from build123d import *

# Parameters (mm, degrees)
SKETCH_1_W      = 23
SKETCH_1_H      = 20
SKETCH_1_R      = 0.5
SKETCH_1_R_2    = 1.5
EXTRUDE_1_DEPTH = 2
SKETCH_2_R      = 3
SKETCH_2_R_2    = 1.5
EXTRUDE_2_DEPTH = 4


with BuildPart() as part:
    # 草图1 → 凸台-拉伸1 (new body)
    with BuildSketch(Plane.XY):
        Rectangle(SKETCH_1_W, SKETCH_1_H)
        with Locations((-8.5, 9)):
            Circle(SKETCH_1_R, mode=Mode.SUBTRACT)
        with Locations((-7.803030303, -9)):
            Circle(SKETCH_1_R, mode=Mode.SUBTRACT)
        with Locations((9.5, 0)):
            Circle(SKETCH_1_R, mode=Mode.SUBTRACT)
        with Locations((2.5, 8)):
            Circle(SKETCH_1_R, mode=Mode.SUBTRACT)
        with Locations((2.5, -8)):
            Circle(SKETCH_1_R, mode=Mode.SUBTRACT)
        with Locations((5.5, 0)):
            Circle(SKETCH_1_R_2, mode=Mode.SUBTRACT)
    extrude(amount=EXTRUDE_1_DEPTH)

    # 草图2 → 凸台-拉伸2 (add)
    with BuildSketch(Plane.XY.offset(2)):
        with Locations((5.5, 0)):
            Circle(SKETCH_2_R)
        with Locations((5.5, 0)):
            Circle(SKETCH_2_R_2, mode=Mode.SUBTRACT)
    extrude(amount=EXTRUDE_2_DEPTH)


solid = part.part
Source: CAD feature listing. Evaluate the final solid. Frame: model axes, mm. Coordinates: 2 decimals unless noted, no trailing zeros. Loops run counter-clockwise (first coordinate to the right, second up) from the corner with the lowest first, then second, coordinate; pieces in that order, holes last. Notation, with made-up numbers: M -38.5,33 L 0.5,33 A16 cw 0.5,56 Z; hole C 87,5 d1. An arc over 180 degrees is marked long. Answer in a Markdown table with one row per item.
Q1. Section A-A on y = 0. Return the cut outline in (x, z).
Answers below:
| item | result |
|---|---|
| outline | M -11.5,0 L 4,0 L 4,6 L 2.5,6 L 2.5,2 L -11.5,2 Z; M 7,0 L 9,0 L 9,2 L 8.5,2 L 8.5,6 L 7,6 Z; M 10,0 L 11.5,0 L 11.5,2 L 10,2 Z |
Q2. Section C-C on y = -9. Return the cut outline in (x, z).
Answers below:
| item | result |
|---|---|
| outline | M -11.5,0 L -8.3,0 L -8.3,2 L -11.5,2 Z; M -7.3,0 L 11.5,0 L 11.5,2 L -7.3,2 Z |
Q3. Section D-D on z = 0.8. Return the cut outline in (x, y).
Answers below:
| item | result |
|---|---|
| outline | M -11.5,-10 L 11.5,-10 L 11.5,10 L -11.5,10 Z; hole C -8.5,9 d1; hole C -7.8,-9 d1; hole C 2.5,-8 d1; hole C 2.5,8 d1; hole C 5.5,0 d3; hole C 9.5,0 d1 |
Q4. First-contact query: pin 1 (2.5 mm diameter, centred on x = 5.5, y = 0, fed in from -Z); pin 2 (3 mm diameter, centred on x = -2, y = -0.5, fed in from +Z). Flat tips, straight axial feed; report the tip coordinate or a pass-through.
Answers below:
| item | result |
|---|---|
| pin 1 | passes through |
| pin 2 | stops at z = 2 |
Q5. Draft query along Y for faces 1 (the cylindrical face through (4.3, -0.9, 3)), 2 (the cylindrical face through (9, 0, 1)), 3 (the flat face through (0, -10, 1)), 4 (the cylindrical face through (8.27, -1.15, 3.97)). Return one class per face: pulls with the +Y half, pulls with the -Y half, needs draft (parallel to the pull), parting line crosses it, or undercut.
Answers below:
| item | result |
|---|---|
| face 1 | undercut |
| face 2 | undercut |
| face 3 | pulls with the -Y half |
| face 4 | parting line crosses it |
Q6. Ray query, probe 1 along Y at (x, z) = (2.5, 1.05); probe 2 along Y at (x, z) = (5.5, 3.1); probe 3 along Z at (x, y) = (-3.5, 2.5). Return the intervals inside material, ascending. Write a range as from..to.
Answers below:
| item | result |
|---|---|
| probe 1 | y = -10..-8.5, -7.5..7.5, 8.5..10 |
| probe 2 | y = -3..-1.5, 1.5..3 |
| probe 3 | z = 0..2 |
Q7. Section B-B on x = 5.5. Return the cut outline in (y, z).
Answers below:
| item | result |
|---|---|
| outline | M -10,0 L -1.5,0 L -1.5,6 L -3,6 L -3,2 L -10,2 Z; M 1.5,0 L 10,0 L 10,2 L 3,2 L 3,6 L 1.5,6 Z |
